from build123d import *

# Parameters (mm, degrees)
SKETCH1_R           = 12.5
BOSS_EXTRUDE1_DEPTH = 1.5
SKETCH2_R           = 3.25
CUT_EXTRUDE1_DEPTH  = 18.741194999
SKETCH3_R           = 4
SKETCH3_R_2         = 3.25
BOSS_EXTRUDE2_DEPTH = 3.5
CUT_EXTRUDE2_START  = -1
SKETCH4_R           = 12.5
SKETCH4_R_2         = 9.875
CUT_EXTRUDE2_DEPTH  = 1
CUT_EXTRUDE3_DEPTH  = 19.241436347
FILLET1_R           = 3.125
FILLET2_R           = 1
SKETCH6_R           = 1.025
CUT_EXTRUDE4_DEPTH  = 19.371173207


with BuildPart() as part:
    # Sketch1 → Boss-Extrude1 (new body)
    with BuildSketch(Plane(origin=(0, 0, 0), x_dir=(1, 0, 0), z_dir=(0, 1, 0))):
        with Locations(Location((0, 0, 0), (0, 0, 270))):
            Circle(SKETCH1_R)
    extrude(amount=BOSS_EXTRUDE1_DEPTH)

    # Sketch2 → Cut-Extrude1 (cut, through all)
    with BuildSketch(Plane.XZ):
        with Locations(Location((0, 0, 0), (0, 0, 270))):
            Circle(SKETCH2_R)
    extrude(amount=-CUT_EXTRUDE1_DEPTH, mode=Mode.SUBTRACT)

    # Sketch3 → Boss-Extrude2 (add)
    with BuildSketch(Plane(origin=(0, 1.5, 0), x_dir=(1, 0, 0), z_dir=(0, 1, 0))):
        with Locations(Location((0, 0, 0), (0, 0, 270))):
            Circle(SKETCH3_R)
        with Locations(Location((0, 0, 0), (0, 0, 90))):
            Circle(SKETCH3_R_2, mode=Mode.SUBTRACT)
    extrude(amount=BOSS_EXTRUDE2_DEPTH)

    # Sketch4 → Cut-Extrude2 (cut)
    with BuildSketch(Plane(origin=(0, 1.5, 0), x_dir=(1, 0, 0), z_dir=(0, 1, 0)).offset(CUT_EXTRUDE2_START)):
        with Locations(Location((0, 0, 0), (0, 0, 270))):
            Circle(SKETCH4_R)
        with Locations(Location((0, 0, 0), (0, 0, 270))):
            Circle(SKETCH4_R_2, mode=Mode.SUBTRACT)
    extrude(amount=CUT_EXTRUDE2_DEPTH, mode=Mode.SUBTRACT)

    # Sketch5 → Cut-Extrude3 (cut, through all)
    with BuildSketch(Plane(origin=(0, 0.5, 0), x_dir=(1, 0, 0), z_dir=(0, 1, 0))):
        with BuildLine():
            ThreePointArc((0, 9.875), (2.96946977, 9.417954889), (5.664067309, 8.089126437))
            Line((5.664067309, 8.089126437), (7.169705454, 10.239400554))
            ThreePointArc((7.169705454, 10.239400554), (3.758822494, 11.921461884), (0, 12.5))
            Line((0, 12.5), (0, 9.875))
        make_face()
        with BuildLine():
            ThreePointArc((-5.664067309, 8.089126437), (-2.96946977, 9.417954889), (0, 9.875))
            Line((0, 9.875), (0, 12.5))
            ThreePointArc((0, 12.5), (-3.758822494, 11.921461884), (-7.169705454, 10.239400554))
            Line((-7.169705454, 10.239400554), (-5.664067309, 8.089126437))
        make_face()
    extrude(amount=-CUT_EXTRUDE3_DEPTH, mode=Mode.SUBTRACT)

    # Fillet1
    # the kernel refuses this fillet: 3.125 mm, written as the material it adds along each edge
    with BuildSketch(Plane(origin=(-5.664067309, 0.5, -8.089126437), x_dir=(-0.5735764363510301, 0, -0.819152044289003), z_dir=(0, -1, 0))) as fillet1_piece_1:
        with BuildLine():
            CenterArc((2.744375, 3.122719105), FILLET1_R, 193.898885593, 73.911882973)
            Line((-0.289128606, 2.372065474), (-0.349798678, 2.357052401))
            ThreePointArc((-0.349798678, 2.357052401), (-0.134589479, 1.187248558), (-0.0625, 0))
            Line((-0.0625, 0), (0, -0.0625))
            ThreePointArc((0, -0.0625), (1.3125, -0.0625), (2.6226125, -0.062454382))
            Line((2.6226125, -0.062454382), (2.625, 0))
        make_face()
    extrude(amount=0.5)
    with BuildSketch(Plane(origin=(5.664067309, 0.5, -8.089126437), x_dir=(-0.8825329923236406, 0, -0.4702504837427398), z_dir=(0, -1, 0))) as fillet1_piece_2:
        with BuildLine():
            CenterArc((2.767725938, 3.102041567), FILLET1_R, 189.13867423, 73.911882973)
            Line((-0.317607894, 2.605714916), (-0.379314571, 2.595788383))
            ThreePointArc((-0.379314571, 2.595788383), (-0.220844779, 1.295295365), (-0.062040831, -0.007562093))
            Line((-0.062040831, -0.007562093), (0.007562093, -0.062040831))
            ThreePointArc((0.007562093, -0.062040831), (1.194810651, 0.010048648), (2.382059209, -0.062040831))
            Line((2.382059209, -0.062040831), (2.389621301, 0))
        make_face()
    extrude(amount=0.5)

    # Fillet2
    fillet2_edges = [part.edges().sort_by_distance(p)[0] for p in [
        (-7.169705454, 0.25, -10.239400554),
        (7.169705454, 0.25, -10.239400554),
    ]]
    fillet(fillet2_edges, radius=FILLET2_R)

    # Sketch6 → Cut-Extrude4 (cut, through all)
    with BuildSketch(Plane.XZ):
        with Locations(Location((-5, 7.125, 0), (0, 0, 270))):
            Circle(SKETCH6_R)
        with Locations(Location((5, 7.125, 0), (0, 0, 270))):
            Circle(SKETCH6_R)
        with Locations(Location((5, -7.125, 0), (0, 0, 270))):
            Circle(SKETCH6_R)
        with Locations(Location((-5, -7.125, 0), (0, 0, 270))):
            Circle(SKETCH6_R)
    extrude(amount=-CUT_EXTRUDE4_DEPTH, mode=Mode.SUBTRACT)


solid = part.part
The model under review builds one solid part; all positions refer to its coordinate system, in mm. A direction names the side the tool comes from. Give positions to 0.01 mm unless a question says otherwise; leave off trailing zeros. Order: outer loops, then holes, each group sorted by start corner. A loop starts at its lowest first (then second) coordinate and runs counter-clockwise, first axis right, second up. Notation, with made-up numbers: M 6.5,62.25 L 51.5,62.25 A29 ccw 51.5,90.25 Z; hole C -34,74 d7. An arc over 180 degrees is marked long. Use one line per item in the form item = value. Start each with the question number.
Item 1: We need section A-A on z = 0. Give the boundary of the cut face in (x, y) (3 decimals), plus the area to 4 significant figures.
Item 2: For faces 4 (the flat face through (1, 0, 4)), 5 (the flat face through (-1, 0.5, 10)), list the 3-axis set-ups (+Z, -Z, +X, -X, +Y, -Y) from which the entire face can be reached by the end or side of a thin tool; tool diameter is ignored.
Item 3: The part is to be moulded in two halves that separate along X. For faces 1 (the flat face through (3, 5, -2)), 2 (the cylindrical face through (4.38, 0.74, -6.31)), 3 (the cylindrical face through (-3.905, 3.226, -0.867)), say which applies: pulls with the +X half, pulls with the -X half, needs draft (parallel to the pull), parting line crosses it, or undercut.
Item 4: We need section D-D on y = 1.1. Give the boundary of the cut face in (x, z) (3 decimals), plus the area to 3 significant figures.
Item 5: To check wall thickness, follow line 1 along X through (y, z) = (2.8, 0); line 2 along X through (y, z) = (1, 7.75); line 3 along Y through (x, z) = (-10, -2.25). State the ranges of each line that lie inside material, in increasing order. Write a range as from..to.
Item 6: Insertion check: pin 1 Ø2.5 at (x, z) = (5, 7.125) entering from -Y; pin 2 Ø1 at (y, z) = (4, 5.5) entering from +X; pin 3 Ø2.5 at (x, z) = (-5, 7.125) entering from +Y; pin 4 Ø1 at (y, z) = (4.5, -4) entering from -X. Each pin has a flat end and moves straight along its axis. Give the tip position at first contact, or say it passes through.
Item 7: We need section C-C on z = 6.75. Give the boundary of the cut face in (x, y).
Item 8: We need section B-B on x = 5. Give the boundary of the cut face in (y, z), plus the area to 3 significant figures.
Completed:
q1.outline = M -12.5,0 L -3.25,0 L -3.25,5 L -4,5 L -4,1.5 L -9.875,1.5 L -9.875,0.5 L -12.5,0.5 Z; M 3.25,0 L 12.5,0 L 12.5,0.5 L 9.875,0.5 L 9.875,1.5 L 4,1.5 L 4,5 L 3.25,5 Z
q1.area = 27.75 mm²
q2.face_4 = +Z, -Z, +X, -X, -Y
q2.face_5 = +Y
q3.face_1 = needs draft
q3.face_2 = undercut
q3.face_3 = parting line crosses it
q4.outline = C 0,0 d19.75; hole C -5,-7.125 d2.05; hole C -5,7.125 d2.05; hole C 0,0 d6.5; hole C 5,-7.125 d2.05; hole C 5,7.125 d2.05
q4.area = 260 mm²
q5.line_1 = -4..-3.25, 3.25..4
q5.line_2 = -6.12..-5.81, -4.19..4.19, 5.81..6.12
q5.line_3 = 0..0.5
q6.pin_1 = 0
q6.pin_2 = through
q6.pin_3 = 1.5
q6.pin_4 = -1.94
q7.outline = M -10.52,0 L -5.95,0 L -5.95,1.5 L -7.21,1.5 L -7.21,0.5 L -10.52,0.5 Z; M -4.05,0 L 4.05,0 L 4.05,1.5 L -4.05,1.5 Z; M 5.95,0 L 10.52,0 L 10.52,0.5 L 7.21,0.5 L 7.21,1.5 L 5.95,1.5 Z
q8.outline = M 0,-9.02 L 0.5,-9.02 L 0.5,-8.52 L 1.5,-8.52 L 1.5,-8.15 L 0,-8.15 Z; M 0,-6.1 L 1.5,-6.1 L 1.5,6.1 L 0,6.1 Z; M 0,8.15 L 1.5,8.15 L 1.5,8.52 L 0.5,8.52 L 0.5,11.46 L 0,11.46 Z
q8.area = 21.1 mm²
